Design review of the part built by this model. Coordinates are the model's own, in mm. A direction names the side the tool comes from. Coordinates: 2 decimals unless noted, no trailing zeros. Write each loop counter-clockwise with the first axis right and the second up, starting at its lowest first coordinate (ties: lowest second). Pieces come first, ordered by that corner, then holes. Notation, with made-up numbers: M 44,53.5 L 53,53.5 A33 ccw 53,90.5 Z; hole C 86,-17.75 d3. An arc over 180 degrees is marked long. One line per question, with ' | ' between items.
Autodesk Fusion 360 part; units mm, degrees
sketch "Sketch1" plane through (0, 0, 0) normal (0, 0, 1) x (1, 0, 0)
  line L0 (32.8868, 25) -> (35.7735, 30)
  line L1 (35.7735, 30) -> (32.8868, 35)
  line L2 (32.8868, 35) -> (27.1132, 35)
  line L3 (27.1132, 35) -> (24.2265, 30)
  line L4 (24.2265, 30) -> (27.1132, 25)
  line L5 (27.1132, 25) -> (32.8868, 25)
  point P0 (30, 30)
  dimension "d1" = 5
extrude "Extrude1" add sketch "Sketch1" along normal blind 80
hole "Hole1" at (29.7914, 30.1949, 0) direction (0, 0, 1) diameter 3.332 depth 6 tip angle 180
hole "Hole2" at (30, 29.7466, 80) direction (0, 0, -1) diameter 3.332 depth 6 tip angle 180
1. Insertion check: pin 1 Ø1 at (x, y) = (29.5, 30.5) entering from -Z; pin 2 Ø2 at (y, z) = (32, 48.5) entering from -X. Each pin has a flat end and moves straight along its axis. Give the tip position at first contact, or say it passes through.
Answer sheet:
pin 1: z = 6 | pin 2: x = 24.8
2. Draft analysis for pull direction X (two halves, no side actions). For faces 1 (the face through (31.2, 29, 0)), 2 (the face through (31.418, 29.834, 3.042)), 3 (the face through (30, 30, 6)), 4 (the face through (25.69, 32.535, 39.44)), state which applies: pulls with the +X half, pulls with the -X half, needs draft (parallel to the pull), parting line crosses it, or undercut.
Answer sheet:
face 1: needs draft | face 2: undercut | face 3: undercut | face 4: pulls with the -X half
3. Tool access review of faces 5 (the face through (34.31, 27.465, 39.44)), 6 (the face through (30, 30, 74)): name each direction out of +Z, -Z, +X, -X, +Y, -Y from which nothing blocks a thin tool from reaching the whole face with its end or side.
Answer sheet:
face 5: +Z, -Z, +X, -Y | face 6: +Z
4. To check wall thickness, follow line 1 along Z through (x, y) = (30.25, 28.75); line 2 along Y through (x, z) = (34.25, 17); line 3 along X through (y, z) = (30.5, 46). State the ranges of each line that lie inside material, in increasing order. Write a range as [from, to].
Answer sheet:
line 1: [6, 74] | line 2: [27.36, 32.64] | line 3: [24.52, 35.48]
5. Take a section at B-B (x = 29). Write out the cut boundary in (y, z), then the cut area to 3 significant figures.
Answer sheet:
outline: M 25,0 L 28.73,0 L 28.73,6 L 31.66,6 L 31.66,0 L 35,0 L 35,80 L 31.08,80 L 31.08,74 L 28.41,74 L 28.41,80 L 25,80 Z | area: 766 mm^2
6. Take a section at C-C (x = 34). Write out the cut boundary in (y, z).
Answer sheet:
outline: M 26.93,0 L 33.07,0 L 33.07,80 L 26.93,80 Z
7. Take a section at A-A (z = 8). Write out the cut boundary in (x, y).
Answer sheet:
outline: M 24.23,30 L 27.11,25 L 32.89,25 L 35.77,30 L 32.89,35 L 27.11,35 Z
